from build123d import *

# Parameters (mm, degrees)
SKETCH1_R           = 3
SKETCH1_R_2         = 1
BOSS_EXTRUDE1_DEPTH = 2
SKETCH2_R           = 0.5
CUT_EXTRUDE1_DEPTH  = 0.5


with BuildPart() as part:
    # Sketch1 → Boss-Extrude1 (new body)
    with BuildSketch(Plane.XY):
        with BuildLine():
            Line((-8.642138301, 3), (8.642138301, 3))
            ThreePointArc((8.642138301, 3), (10.578686732, 2.291239877), (11.600202961, 0.49985345))
            ThreePointArc((11.600202961, 0.49985345), (14.900135896, -10.538397729), (6.187782244, -3))
            Line((6.187782244, -3), (-6.187782244, -3))
            ThreePointArc((-6.187782244, -3), (-14.900135896, -10.538397729), (-11.600202961, 0.49985345))
            ThreePointArc((-11.600202961, 0.49985345), (-10.578686732, 2.291239877), (-8.642138301, 3))
        make_face()
        with Locations((-11.642138301, -5.5)):
            Circle(SKETCH1_R, mode=Mode.SUBTRACT)
        with Locations((11.642138301, -5.5)):
            Circle(SKETCH1_R, mode=Mode.SUBTRACT)
        with Locations((8.642138301, 0)):
            Circle(SKETCH1_R_2, mode=Mode.SUBTRACT)
        with Locations((-8.642138301, 0)):
            Circle(SKETCH1_R_2, mode=Mode.SUBTRACT)
        Circle(SKETCH1_R_2, mode=Mode.SUBTRACT)
    extrude(amount=BOSS_EXTRUDE1_DEPTH)

    # Sketch2 → Cut-Extrude1 (cut)
    with BuildSketch(Plane.XZ.offset(3)):
        with Locations((0, 1)):
            Circle(SKETCH2_R)
    extrude(amount=-CUT_EXTRUDE1_DEPTH, mode=Mode.SUBTRACT)


solid = part.part
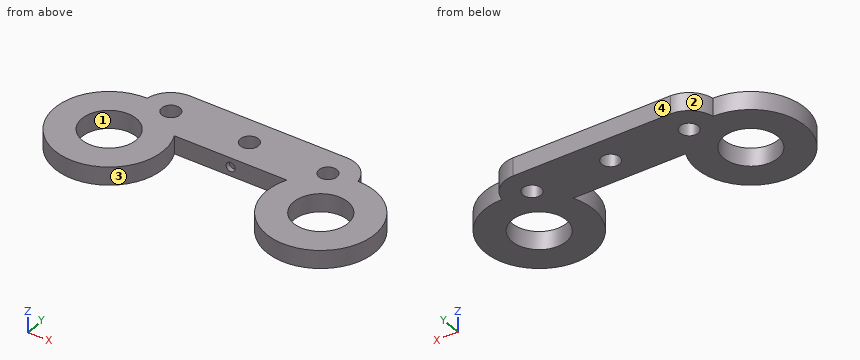
Model file for the job. Use its own axes, mm. Face numbers are marked on the shaded views. Give positions to 0.01 mm unless a question says otherwise; leave off trailing zeros. Write each loop counter-clockwise with the first axis right and the second up, starting at its lowest first coordinate (ties: lowest second). Pieces come first, ordered by that corner, then holes. Notation, with made-up numbers: (22, 86.25) -> (32, 86.25) arc R22 cw to (32, 110.25) -> close; hole circle Ø4 at (2, 67). An arc over 180 degrees is marked (long way). Write item = value, one per line.
(1) Slice it at D-D, the plane x = -14. Give the cut face in (y, z).
Determined:
outline = (-11.02, 0) -> (-7.35, 0) -> (-7.35, 2) -> (-11.02, 2) -> close; (-3.65, 0) -> (0.02, 0) -> (0.02, 2) -> (-3.65, 2) -> close
(2) Flat gauge pin, fed straight in: P1, Ø0.5, axis at x = 0, z = 1, coming from the -Y side. Where does the tip first touch, or does it go through?
Determined:
P1 = -2.5
(3) Probe line 1 along X through (y, z) = (0.75, 1.7); line 2 along X through (y, z) = (-8.25, 0.8); line 3 along Y through (x, z) = (0, 1.45). List the from-to ranges inside material, lowest first.
Determined:
line_1 = -11.55 to -9.3, -7.98 to -0.66, 0.66 to 7.98, 9.3 to 11.55
line_2 = -16.97 to -12.84, -10.44 to -6.31, 6.31 to 10.44, 12.84 to 16.97
line_3 = -2.5 to -1, 1 to 3
(4) Slice it at C-C, the plane y = -9.25. Give the cut face in (x, z), then the cut area to 3 significant figures.
Determined:
outline = (-16.33, 0) -> (-6.96, 0) -> (-6.96, 2) -> (-16.33, 2) -> close; (6.96, 0) -> (16.33, 0) -> (16.33, 2) -> (6.96, 2) -> close
area = 37.5 mm2
(5) Mould opens along X. For the marked faces 1, 2, 3 and 4 say: released by +X, released by -X, zero draft, split by the parting line, or undercut.
Determined:
face_1 = undercut
face_2 = released by -X
face_3 = undercut
face_4 = zero draft
(6) Slice it at B-B, the plane y = -5.5. Give the cut face in (x, z), then the cut area to 3 significant figures.
Determined:
outline = (-17.64, 0) -> (-14.64, 0) -> (-14.64, 2) -> (-17.64, 2) -> close; (-8.64, 0) -> (-5.64, 0) -> (-5.64, 2) -> (-8.64, 2) -> close; (5.64, 0) -> (8.64, 0) -> (8.64, 2) -> (5.64, 2) -> close; (14.64, 0) -> (17.64, 0) -> (17.64, 2) -> (14.64, 2) -> close
area = 24.0 mm2
(7) Slice it at A-A, the plane x = 0. Give the cut face in (y, z).
Determined:
outline = (-3, 0) -> (-1, 0) -> (-1, 2) -> (-3, 2) -> (-3, 1.5) -> (-2.5, 1.5) -> (-2.5, 0.5) -> (-3, 0.5) -> close; (1, 0) -> (3, 0) -> (3, 2) -> (1, 2) -> close
